```python
from build123d import *

# Parameters (mm, degrees)
F1_DEPTH = 17.5
F2_R     = 4
F3_DEPTH = 25
F4_R     = 4.4
F5_DEPTH = 25
F6_R     = 2


# Not quite as in the source:
# - a feature names something its author has since deleted; it is built from what else it names


with BuildPart() as f1:
    # F0 (on Front) → F1 (new body, symmetric)
    with BuildSketch(Plane.XZ):
        Polygon((95, -38), (95, 10), (-95, 10), (-95, -38), (-115, -38), (-115, -40), (-93, -40), (-93, 8), (93, 8), (93, -40), (115, -40), (115, -38), align=None)
    extrude(amount=F1_DEPTH, both=True)

    # F2 (on face) → F3 (cut)
    with BuildSketch(Plane.XY.offset(-38)):
        with Locations((-105, 0)):
            Circle(F2_R)
        with Locations((105, 0)):
            Circle(F2_R)
    extrude(amount=-F3_DEPTH, mode=Mode.SUBTRACT)

    # F4 (on face) → F5 (cut)
    with BuildSketch(Plane.XY.offset(10)):
        with Locations((-32.5, 0)):
            Circle(F4_R)
        with Locations((32.5, 0)):
            Circle(F4_R)
    extrude(amount=-F5_DEPTH, mode=Mode.SUBTRACT)

    # F6
    f6_edges = [f1.edges().sort_by_distance(p)[0] for p in [
        (95, 0, 10),
        (-95, 0, 10),
        (-93, 0, -40),
        (93, 0, -40),
    ]]
    fillet(f6_edges, radius=F6_R)


solid = f1.part
```
Could you check a few things on this model? Use its own coordinates, in mm. A direction names the side the tool comes from. Give positions to 0.01 mm unless a question says otherwise; leave off trailing zeros. Order: outer loops, then holes, each group sorted by start corner. A loop starts at its lowest first (then second) coordinate and runs counter-clockwise, first axis right, second up.
Q1. For faces 4 (the flat face through (95, 0, -15)), 5 (the flat face through (-1, 0, 8)), 6 (the flat face through (-107, -4, -38)), which set-ups out of +Z, -Z, +X, -X, +Y, -Y let a thin tool reach every point of the face, with its end or its side?
Q2. Suppose I cut it at B-B, the plane x = 105. Write out the boundary of the cut face in (y, z).
Q3. We'd pull the mould along Y, two halves only. Please class faces 1 (the flat face through (-1, -17.5, 9)), 2 (the cylindrical face through (36.564, -1.685, 9.014)), 3 (the flat face through (1, 0, 10)): +Y half, -Y half, draft (parallel to the pull), parting line (faces both ways), or undercut.
Q4. Suppose I cut it at A-A, the plane z = 0. Write out the boundary of the cut face in (x, y), and give its area (3 significant figures).
Q5. Suppose I cut it at C-C, the plane y = 10. Write out the boundary of the cut face in (x, z), and give its area (3 significant figures).
Q6. I'm going to push flat-ended pins straight in: P1, Ø1, axis at y = 4.5, z = -27.5, coming from the +X side; P2, Ø17.5, axis at y = 5, z = -4, coming from the -X side; P3, Ø6, axis at x = 66.5, y = -4, coming from the -Z side; P4, Ø10.5, axis at x = 105, y = 0, coming from the -Z side. Where does each tip first touch, or does it pass through?
Q7. Suppose I cut it at D-D, the plane x = -83.5. Write out the boundary of the cut face in (y, z).
Q8. If I drill on line 1 along Y through (x, z) = (32.5, 8.6); line 2 along X through (y, z) = (-11.5, -32); line 3 along Z through (x, y) = (10.5, -14), over which ranges is the centre line in solid material (lowest first)?
Solution:
1. face 4: +Z, +X, +Y, -Y
1. face 5: -Z, +Y, -Y
1. face 6: +Z, -X, +Y, -Y
2. outline: (-17.5, -40) - (-4, -40) - (-4, -38) - (-17.5, -38) - close; (4, -40) - (17.5, -40) - (17.5, -38) - (4, -38) - close
3. face 1: -Y half
3. face 2: undercut
3. face 3: draft
4. outline: (-95, -17.5) - (-93, -17.5) - (-93, 17.5) - (-95, 17.5) - close; (93, -17.5) - (95, -17.5) - (95, 17.5) - (93, 17.5) - close
4. area: 140 mm2
5. outline: (-115, -40) - (-95, -40) arc R2 ccw to (-93, -38) - (-93, 8) - (93, 8) - (93, -38) arc R2 ccw to (95, -40) - (115, -40) - (115, -38) - (95, -38) - (95, 8) arc R2 ccw to (93, 10) - (-93, 10) arc R2 ccw to (-95, 8) - (-95, -38) - (-115, -38) - close
5. area: 649 mm2
6. P1: stops at x = 95
6. P2: stops at x = -95
6. P3: stops at z = 8
6. P4: stops at z = -40
7. outline: (-17.5, 8) - (17.5, 8) - (17.5, 10) - (-17.5, 10) - close
8. line 1: y = -17.5 to -4.4, 4.4 to 17.5
8. line 2: x = -95 to -93, 93 to 95
8. line 3: z = 8 to 10
